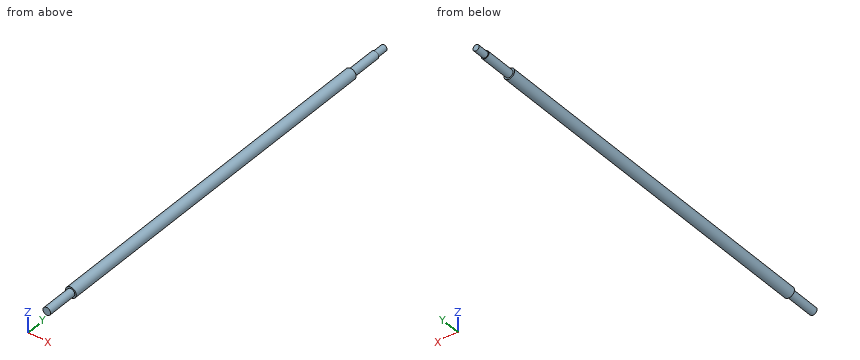
Autodesk Inventor part; units mm, degrees
ref_plane "YZ Plane" through (0, 0, 0) normal (1, 0, 0) x (0, 1, 0)
ref_plane "XZ Plane" through (0, 0, 0) normal (0, 1, 0) x (-1, 0, 0)
ref_plane "XY Plane" through (0, 0, 0) normal (0, 0, 1) x (1, 0, 0)
sketch "Sketch1" plane through (0, 0, 0) normal (0, 1, 0) x (-1, 0, 0)
  circle A0 centre (0, 0) radius 7
  dimension "d0" = 14
extrude "Extrusion1" add sketch "Sketch1" along normal mid plane 464
sketch "Sketch2" plane through (0, 232, 0) normal (0, 1, 0) x (1, 0, 0)
  circle A0 centre (0, 0) radius 5
  dimension "d3" = 10
extrude "Extrusion2" add sketch "Sketch2" along normal blind 40
sketch "Sketch3" plane through (0, 272, 0) normal (0, 1, 0) x (1, 0, 0)
  circle A0 centre (0, 0) radius 4
  dimension "d6" = 8
extrude "Extrusion3" add sketch "Sketch3" along normal blind 15
thread "Thread1"
sketch "Sketch4" plane through (0, -232, 0) normal (0, -1, 0) x (1, 0, 0)
  circle A0 centre (0, 0) radius 5
  circle A1 centre (0, 0) radius 5
  dimension "d13" = 10
extrude "Extrusion4" add sketch "Sketch4" along normal blind 40
properties part number "Screw Replica"
Here's how the part is built. I have some questions about the finished solid (model axes, mm). Give positions to 0.01 mm unless a question says otherwise; leave off trailing zeros. Write each loop counter-clockwise with the first axis right and the second up, starting at its lowest first coordinate (ties: lowest second). Pieces come first, ordered by that corner, then holes. Notation, with made-up numbers: (-37, -10) -> (-30, -10) arc R23 cw to (-30, 12) -> close; hole circle Ø6 at (39, -12.5). An arc over 180 degrees is marked (long way). Use one line per item in the form item = value.
1) I'm going to push a flat-ended pin straight in: pin 1 (5 mm diameter, centred on y = -188.5, z = 3, fed in from -X). Where does the tip first touch, or does it pass through?
Verdict:
pin_1 = -6.98
2) Suppose I cut it at B-B (z = 0). Please give me the cut outline in (x, y).
Verdict:
outline = (-7, -232) -> (-5, -232) -> (-5, -272) -> (5, -272) -> (5, -232) -> (7, -232) -> (7, 232) -> (5, 232) -> (5, 272) -> (4, 272) -> (4, 287) -> (-4, 287) -> (-4, 272) -> (-5, 272) -> (-5, 232) -> (-7, 232) -> close
3) Suppose I cut it at A-A (x = 0). Please give me the cut outline in (y, z), and give its area (3 significant figures).
Verdict:
outline = (-272, -5) -> (-232, -5) -> (-232, -7) -> (232, -7) -> (232, -5) -> (272, -5) -> (272, -4) -> (287, -4) -> (287, 4) -> (272, 4) -> (272, 5) -> (232, 5) -> (232, 7) -> (-232, 7) -> (-232, 5) -> (-272, 5) -> close
area = 7,420 mm2
4) If I drill on L1, parallel to Y at x = -6.25, z = 0; L2, parallel to X at y = -205, z = 5.75; L3, parallel to X at y = -236, z = 0.5, over which ranges is the centre line in solid material (lowest first)? Write a range as [from, to].
Verdict:
L1 = [-232, 232]
L2 = [-3.99, 3.99]
L3 = [-4.97, 4.97]
5) Suppose I cut it at C-C (y = 94). Please give me the cut outline in (x, z).
Verdict:
outline = circle Ø14 at (0, 0)
